Geometry check sheet. Reference: the model listing, model coordinates, mm. A direction names the side the tool comes from. Give positions to 0.01 mm unless a question says otherwise; leave off trailing zeros. Write each loop counter-clockwise with the first axis right and the second up, starting at its lowest first coordinate (ties: lowest second). Pieces come first, ordered by that corner, then holes. Notation, with made-up numbers: M 48,82 L 90,82 A13 ccw 90,102 Z; hole C 17.5,33.5 d7. An arc over 180 degrees is marked long. Use one line per item in the form item = value. Start each with the question number.
```python
from build123d import *

# Parameters (mm, degrees)
SKETCH1_R           = 14
BOSS_EXTRUDE1_DEPTH = 38
CUT_EXTRUDE1_START  = 8
SKETCH2_W           = 2
SKETCH2_H           = 3
CUT_EXTRUDE1_DEPTH  = 20


with BuildPart() as part:
    # Sketch1 → Boss-Extrude1 (new body)
    with BuildSketch(Plane(origin=(0, 0, 0), x_dir=(1, 0, 0), z_dir=(0, 1, 0))):
        Circle(SKETCH1_R)
    extrude(amount=BOSS_EXTRUDE1_DEPTH)

    # Sketch2 → Cut-Extrude1 (cut)
    with BuildSketch(Plane(origin=(0, 0, 0), x_dir=(1, 0, 0), z_dir=(0, 1, 0)).offset(CUT_EXTRUDE1_START)):
        with Locations((0, -13.5)):
            Rectangle(SKETCH2_W, SKETCH2_H)
    extrude(amount=CUT_EXTRUDE1_DEPTH, mode=Mode.SUBTRACT)


solid = part.part
```
(1) Sectioned sample at C-C, the plane z = -7.25. Record the boundary of the cut face in (x, y).
(2) Depth check by flat-ended pin: pin 1 (1.6 mm diameter, centred on x = 0.5, y = 14, fed in from +Z); pin 2 (3 mm diameter, centred on y = 8.5, z = -2.5, fed in from +X); pin 3 (0.6 mm diameter, centred on y = 15.5, z = 13, fed in from +X). Enter the tip coordinate at first touch or a pass-through.
(3) Sectioned sample at A-A, the plane x = 0. Record the boundary of the cut face in (y, z).
(4) Thickness scan on probe 1 along X at (y, z) = (24, -0.5); probe 2 along Z at (x, y) = (-5.5, 26.5). Record the ranges inside material, lowest first. Write a range as [from, to].
(5) Sectioned sample at B-B, the plane y = 23.5. Record the boundary of the cut face in (x, z).
(6) Tool access check on faces 1 (the cylindrical face through (12.932, 18.734, 5.362)), 2 (the flat face through (0, 28, 13)). Record the directions out of +Z, -Z, +X, -X, +Y, -Y that give a thin tool (end or side, any length) a straight path to the whole face; none if there is none.
(7) Draft check along Y on faces 3 (the flat face through (0, 0, 0)), 4 (the flat face through (-1, 18, 13)), 5 (the flat face through (0, 38, 0)). Enter one of: released by +Y, released by -Y, zero draft, split by the parting line, or undercut.
(8) Sectioned sample at D-D, the plane y = 33. Record the boundary of the cut face in (x, z), plus the area to 3 significant figures.
Numbers:
q1.outline = M -11.98,0 L 11.98,0 L 11.98,38 L -11.98,38 Z
q2.pin_1 = 13.96
q2.pin_2 = 13.96
q2.pin_3 = 5.89
q3.outline = M 0,-14 L 38,-14 L 38,14 L 28,14 L 28,12 L 8,12 L 8,14 L 0,14 Z
q4.probe_1 = [-13.99, 13.99]
q4.probe_2 = [-12.87, 12.87]
q5.outline = M -1,12 L -1,13.96 A14 ccw long 1,13.96 L 1,12 Z
q6.face_1 = +Y, -Y
q6.face_2 = +Z
q7.face_3 = released by -Y
q7.face_4 = undercut
q7.face_5 = released by +Y
q8.outline = C 0,0 d28
q8.area = 616 mm2
